Source: three-view drawing plus pictorial views. Frame: mm from the lowest corner of the part. A direction names the side the tool comes from. Coordinates: 2 decimals unless noted, no trailing zeros. Loops run counter-clockwise (first coordinate to the right, second up) from the corner with the lowest first, then second, coordinate; pieces in that order, holes last.
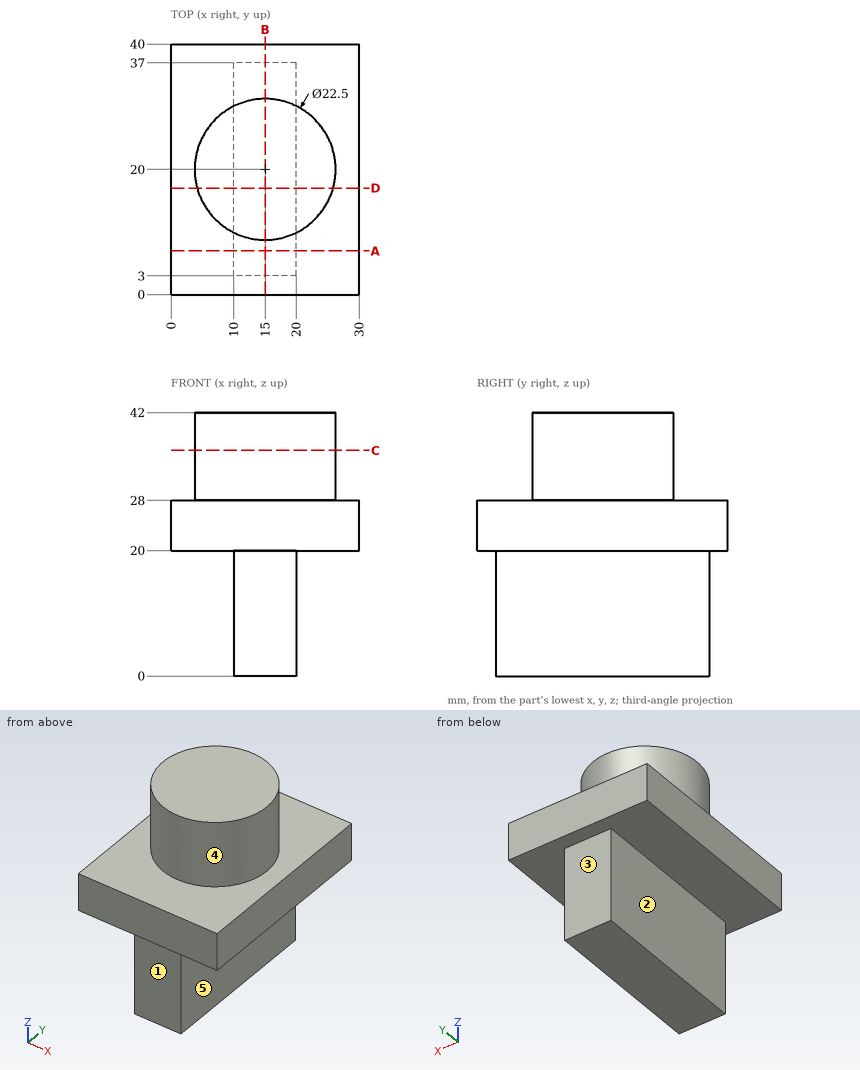
Q1. First-contact query: pin 1 Ø1.5 at (x, z) = (23, 31) entering from +Y; pin 2 Ø3 at (x, z) = (16.5, 14) entering from -Y; pin 3 Ø5 at (y, z) = (16.5, 5) entering from +X. Flat tips, straight axial feed; report the tip coordinate or a pass-through.
Q2. Section query D-D on y = 17. Return the cut outline in (x, z).
Q3. Material intervals for line 1 along Z through (x, y) = (7, 17); line 2 along Z through (x, y) = (26.25, 37); line 3 along X through (y, z) = (4.5, 7), sorted ascending.
Q4. Reachability of the marked faces 1, 2, 3, 4 and 5 from +Z, -Z, +X, -X, +Y, -Y: full face, straight path, thin tool, end or side. Return the list, or none.
Q5. Section query C-C on z = 36. Return the cut outline in (x, y).
Q6. Section query B-B on x = 15. Return the cut outline in (y, z), then the cut area to 4 significant figures.
Q7. Section query A-A on y = 7. Return the cut outline in (x, z), then the cut area to 3 significant figures.
Resolved:
1. pin 1: stops at y = 28.6
1. pin 2: stops at y = 3
1. pin 3: stops at x = 20
2. outline: (0, 20) - (10, 20) - (10, 0) - (20, 0) - (20, 20) - (30, 20) - (30, 28) - (25.84, 28) - (25.84, 42) - (4.16, 42) - (4.16, 28) - (0, 28) - close
3. line 1: z = 20 to 42
3. line 2: z = 20 to 28
3. line 3: x = 10 to 20
4. face 1: -Z, +X, -X, -Y
4. face 2: -Z, -X, +Y, -Y
4. face 3: -Z, +X, -X, +Y
4. face 4: +Z
4. face 5: -Z, +X, +Y, -Y
5. outline: circle Ø22.5 at (15, 20)
6. outline: (0, 20) - (3, 20) - (3, 0) - (37, 0) - (37, 20) - (40, 20) - (40, 28) - (31.25, 28) - (31.25, 42) - (8.75, 42) - (8.75, 28) - (0, 28) - close
6. area: 1,315 mm2
7. outline: (0, 20) - (10, 20) - (10, 0) - (20, 0) - (20, 20) - (30, 20) - (30, 28) - (0, 28) - close
7. area: 440 mm2
